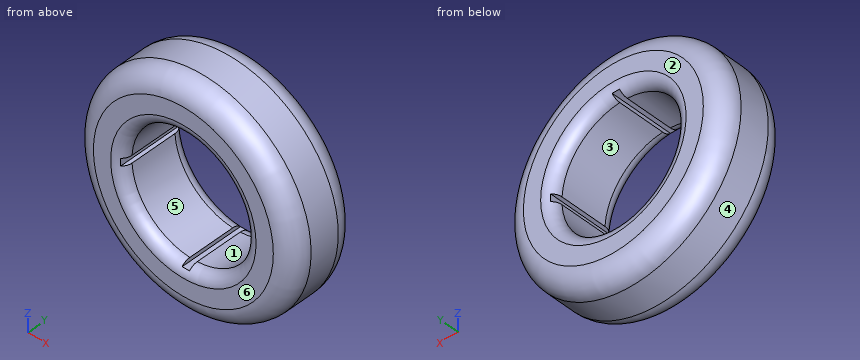
```python
from build123d import *

# Parameters (mm, degrees)
BOX357_W          = 53
BOX357_H          = 30
BOX357_DEPTH      = 3
BOX358_W          = 3
BOX358_H          = 30
BOX358_DEPTH      = 53
CYLINDER020_R     = 25
CYLINDER020_DEPTH = 28
CYLINDER018_R     = 44.5
CYLINDER018_DEPTH = 28
FILLET007_R       = 8
FILLET009_R       = 4.5


with BuildPart() as cube357:
    # Box357 → Box357 (new body)
    with BuildSketch(Plane(origin=(-26.5, 1, -1.5), x_dir=(1, 0, 0), z_dir=(0, 0, 1))):
        with Locations((26.5, 15)):
            Rectangle(BOX357_W, BOX357_H)
    extrude(amount=BOX357_DEPTH)


with BuildPart() as fusion013:
    # Box358 → Box358 (new body)
    with BuildSketch(Plane(origin=(-1.5, 1, -26.5), x_dir=(1, 0, 0), z_dir=(0, 0, 1))):
        with Locations((1.5, 15)):
            Rectangle(BOX358_W, BOX358_H)
    extrude(amount=BOX358_DEPTH)

    # Fusion013: union Cube357
    add(cube357.part)


with BuildPart() as cylinder020:
    # Cylinder020 → Cylinder020 (new body)
    with BuildSketch(Plane(origin=(0, 0, 0), x_dir=(1, 0, 0), z_dir=(0, 1, 0))):
        Circle(CYLINDER020_R)
    extrude(amount=CYLINDER020_DEPTH)


with BuildPart() as rear_wheel_inner:
    # Cylinder018 → Cylinder018 (new body)
    with BuildSketch(Plane(origin=(0, 0, 0), x_dir=(1, 0, 0), z_dir=(0, 1, 0))):
        Circle(CYLINDER018_R)
    extrude(amount=CYLINDER018_DEPTH)

    # Fillet007
    fillet007_edges = [rear_wheel_inner.edges().sort_by_distance(p)[0] for p in [
        (-44.5, 0, 0),
        (-44.5, 28, 0),
    ]]
    fillet(fillet007_edges, radius=FILLET007_R)

    # Cut004026018020018: cut Cylinder020
    add(cylinder020.part, mode=Mode.SUBTRACT)

    # Fillet009
    fillet009_edges = [rear_wheel_inner.edges().sort_by_distance(p)[0] for p in [
        (-25, 28, 0),
        (-25, 0, 0),
    ]]
    fillet(fillet009_edges, radius=FILLET009_R)

    # Cut004026018020019: cut Fusion013
    add(fusion013.part, mode=Mode.SUBTRACT)


solid = rear_wheel_inner.part
```
Geometry: final body of the model. Coordinates: model frame, mm. Face numbers are marked on the shaded views. A direction names the side the tool comes from. Coordinates: 2 decimals unless noted, no trailing zeros. Order: outer loops, then holes, each group sorted by start corner. A loop starts at its lowest first (then second) coordinate and runs counter-clockwise, first axis right, second up. Notation, with made-up numbers: (54, -21) -> (60, -21) arc R18 ccw to (60, -3) -> close; hole circle Ø11 at (67.5, 51). An arc over 180 degrees is marked (long way). Write each question's results on one line, items separated by ' | '. Start each with the question number.
1) Material intervals for line 1 along Z through (x, y) = (-1, 8); line 2 along X through (y, z) = (16.5, -8) (3 decimals); line 3 along X through (y, z) = (4.75, -13), sorted ascending.
2) Mould query, pull axis Z, two halves, no side actions, for the marked faces 1, 2, 3 and 4. Classes: released by +Z, released by -Z, zero draft, split by the parting line, or undercut.
3) Cut plane B-B, the plane z = 0. Output: boundary loops of the cut face in (x, y), and give its area (3 significant figures).
4) Set-up query: the marked faces 5 and 6. Return all of +Z, -Z, +X, -X, +Y, -Y with unobstructed straight access to the full face (end or side cutting, diameter ignored); none if empty.
5) Cut plane C-C, the plane x = 0. Output: boundary loops of the cut face in (y, z).
6) First-contact query: pin 1 (0.5 mm diameter, centred on x = 26, y = 17.5, fed in from +Z); pin 2 (1.7 mm diameter, centred on x = -25.5, y = 8, fed in from -Z); pin 3 (0.8 mm diameter, centred on y = 20, z = 26, fed in from +X); pin 4 (1.5 mm diameter, centred on y = 11, z = -0.5, fed in from -X). Flat tips, straight axial feed; report the tip coordinate or a pass-through.
7) Cut plane A-A, the plane y = 13.75. Output: boundary loops of the cut face in (x, z), and give its area (3 significant figures).
Checks:
1) line 1: -44.49 to -26.5, 26.5 to 44.49 | line 2: -43.775 to -23.685, 23.685 to 43.775 | line 3: -41.84 to -21.35, 21.35 to 41.84
2) face 1: undercut | face 2: zero draft | face 3: undercut | face 4: split by the parting line
3) outline: (-44.5, 8) arc R8 ccw to (-36.5, 0) -> (-29.5, 0) arc R4.5 ccw to (-26.5, 1.15) -> (-26.5, 26.85) arc R4.5 ccw to (-29.5, 28) -> (-36.5, 28) arc R8 ccw to (-44.5, 20) -> close; (26.5, 1.15) arc R4.5 ccw to (29.5, 0) -> (36.5, 0) arc R8 ccw to (44.5, 8) -> (44.5, 20) arc R8 ccw to (36.5, 28) -> (29.5, 28) arc R4.5 ccw to (26.5, 26.85) -> close | area: 949 mm^2
4) face 5: +Y, -Y | face 6: +Z, -Z, +X, -X, -Y
5) outline: (0, -36.5) arc R8 ccw to (8, -44.5) -> (20, -44.5) arc R8 ccw to (28, -36.5) -> (28, -29.5) arc R4.5 ccw to (26.85, -26.5) -> (1.15, -26.5) arc R4.5 ccw to (0, -29.5) -> close; (0, 29.5) arc R4.5 ccw to (1.15, 26.5) -> (26.85, 26.5) arc R4.5 ccw to (28, 29.5) -> (28, 36.5) arc R8 ccw to (20, 44.5) -> (8, 44.5) arc R8 ccw to (0, 36.5) -> close
6) pin 1: z = 36.29 | pin 2: z = -37.05 | pin 3: x = 36.4 | pin 4: x = -44.5
7) outline: circle Ø89 at (0, 0); hole (-26.5, -1.5) -> (-24.95, -1.5) arc R25 ccw to (-1.5, -24.95) -> (-1.5, -26.5) -> (1.5, -26.5) -> (1.5, -24.95) arc R25 ccw to (24.95, -1.5) -> (26.5, -1.5) -> (26.5, 1.5) -> (24.95, 1.5) arc R25 ccw to (1.5, 24.95) -> (1.5, 26.5) -> (-1.5, 26.5) -> (-1.5, 24.95) arc R25 ccw to (-24.95, 1.5) -> (-26.5, 1.5) -> close | area: 4,240 mm^2
